from build123d import *

# Parameters (mm, degrees)
F1_DEPTH  = 12
F3_DEPTH  = 25
F4_R      = 1.6
F5_DEPTH  = 12.001
F4_R_2    = 3.25
F6_DEPTH  = 2.5
F8_DEPTH  = 2.5
F9_R      = 1.65
F10_DEPTH = 34.5196429053
F11_R     = 4.99999


# Not quite as in the source:
# - a fillet or chamfer is up to 0.001 mm smaller than in the source, because OpenCascade refuses the exact size


with BuildPart() as f1:
    # F0 (on Right) → F1 (new body)
    with BuildSketch(Plane.YZ):
        Polygon((-19, 5), (-19, -5), (19, -5), (10.3397459622, 0), (14.535244118, 5), align=None)
        Polygon((10.3397459622, 0), (19, -5), (19, 5), (14.535244118, 5), align=None)
        Polygon((19, 5), (19, -5), (41.5633217274, 32.5436371113), (51.2051358727, 44.0343037581), (48.9070025433, 45.9626665871), (14.535244118, 5), align=None)
    extrude(amount=F1_DEPTH)

    # F2 (on face) → F3 (cut)
    with BuildSketch(Plane.XY.offset(5)):
        with BuildLine():
            ThreePointArc((8.4, -10.2369316877), (8.6239283527, -9.6363961031), (8.7, -9))
            ThreePointArc((8.7, -9), (5.3636038969, -6.3760716473), (3.6, -10.2369316877))
            Line((3.6, -10.2369316877), (8.4, -10.2369316877))
        make_face()
        with BuildLine():
            Line((8.4, -10.2369316877), (3.6, -10.2369316877))
            ThreePointArc((3.6, -10.2369316877), (6, -11.7), (8.4, -10.2369316877))
        make_face()
        with BuildLine():
            ThreePointArc((8.4, -10.2369316877), (6, -11.7), (3.6, -10.2369316877))
            Line((3.6, -10.2369316877), (3.6, -19))
            Line((3.6, -19), (8.4, -19))
            Line((8.4, -19), (8.4, -10.2369316877))
        make_face()
    extrude(amount=-F3_DEPTH, mode=Mode.SUBTRACT)

    # F4 (on face) → F5 (cut, through all)
    with BuildSketch(Plane.YZ.offset(12)):
        with Locations((-14, 0)):
            Circle(F4_R)
    extrude(amount=-F5_DEPTH, mode=Mode.SUBTRACT)

    # F4 (on face) → F6 (cut)
    with BuildSketch(Plane.YZ.offset(12)):
        with Locations((-14, 0)):
            Circle(F4_R_2)
        with Locations((-14, 0)):
            Circle(F4_R, mode=Mode.SUBTRACT)
    extrude(amount=-F6_DEPTH, mode=Mode.SUBTRACT)

    # F7 (on face) → F8 (cut)
    with BuildSketch(Plane(origin=(0, 0, 0), x_dir=(0, -1, 0), z_dir=(-1, 0, 0))):
        Polygon((11.15, 1.6454482672), (11.15, -1.6454482672), (14, -3.2908965344), (16.85, -1.6454482672), (16.85, 1.6454482672), (14, 3.2908965344), align=None)
    extrude(amount=-F8_DEPTH, mode=Mode.SUBTRACT)

    # F9 (on face) → F10 (cut, through all)
    with BuildSketch(Plane(origin=(0, 6.067612003, -5.0913309939), x_dir=(1, 0, 0), z_dir=(0, -0.7660444431, 0.6427876097))):
        with Locations((6, 59.6462605918)):
            Circle(F9_R)
    extrude(amount=-F10_DEPTH, mode=Mode.SUBTRACT)

    # F11 (radius 5 in the source; OpenCascade refuses exactly that, so slightly less here)
    f11_edges = [f1.edges().sort_by_distance(p)[0] for p in [
        (1.8, -19, 5),
        (10.2, -19, 5),
        (1.8, -19, -5),
        (10.2, -19, -5),
        (12, 50.056069, 44.998485),
        (0, 50.056069, 44.998485),
        (6, 14.535244, 5),
        (6, 19, -5),
    ]]
    fillet(f11_edges, radius=F11_R)


solid = f1.part
CAD build for the part. Positions are in the model's coordinates, mm. A direction names the side the tool comes from. Give positions to 0.01 mm unless a question says otherwise; leave off trailing zeros. Order: outer loops, then holes, each group sorted by start corner. A loop starts at its lowest first (then second) coordinate and runs counter-clockwise, first axis right, second up. Notation, with made-up numbers: (39, 76) - (49, 76) arc R14 cw to (49, 103) - close; hole circle Ø3 at (47.5, 87). An arc over 180 degrees is marked (long way). Answer in a Markdown table with one row per item.
1. Probe probe 1 along X at (y, z) = (-9, 2.25); probe 2 along Z at (x, y) = (8.9, -14); probe 3 along Z at (x, y) = (9.75, -3). List the from-to ranges inside material, lowest first. Write a range as [from, to].
Data:
| item | result |
|---|---|
| probe 1 | x = [0, 3.3], [8.7, 12] |
| probe 2 | z = [-5, -1.6], [1.6, 5] |
| probe 3 | z = [-5, 5] |
2. Flat gauge pins, fed straight in: pin 1 (1.2 mm diameter, centred on x = 1.5, z = 1, fed in from +Y); pin 2 (2 mm diameter, centred on y = 43, z = 32, fed in from +X); pin 3 (6 mm diameter, centred on x = 10, z = 28.5, fed in from +Y); pin 4 (5 mm diameter, centred on y = -14, z = 0, fed in from -X). Where does each tip first touch, or does it go through?
Data:
| item | result |
|---|---|
| pin 1 | stops at y = 22.97 |
| pin 2 | passes through |
| pin 3 | stops at y = 40.94 |
| pin 4 | stops at x = 2.5 |
3. Saw through at B-B, the plane y = 26. Give the cut face in (x, z), plus the area to 3 significant figures.
Data:
| item | result |
|---|---|
| outline | (0, 6.65) - (12, 6.65) - (12, 18.66) - (0, 18.66) - close |
| area | 144 mm² |
4. Tool access for faces 1 (the cylindrical face through (10.768, -17.247, 0.143)), 2 (the flat face through (6, -1, 5)), 3 (the flat face through (1.232, -12.595, 2.48)): list every direction of +Z, -Z, +X, -X, +Y, -Y with a clear straight run to the whole face (end or side of a thin tool).
Data:
| item | result |
|---|---|
| face 1 | +X |
| face 2 | +Z, +X, -X, -Y |
| face 3 | -X |
5. Saw through at C-C, the plane z = 20.5. Give the cut face in (x, y).
Data:
| item | result |
|---|---|
| outline | (0, 27.54) - (12, 27.54) - (12, 34.33) - (0, 34.33) - close |
6. Pull direction Z, two halves, no side cores. Call faces 4 (the cylindrical face through (2, -18, 3)), 5 (the flat face through (1.232, -15.405, -2.48)), 6 (the cylindrical face through (10, -17, -4)): pulls with the +Z half, pulls with the -Z half, needs draft (parallel to the pull), parting line crosses it, or undercut.
Data:
| item | result |
|---|---|
| face 4 | pulls with the +Z half |
| face 5 | undercut |
| face 6 | pulls with the -Z half |
7. Saw through at A-A, the plane x = 6. Give the cut face in (y, z).
Data:
| item | result |
|---|---|
| outline | (-6.3, -5) - (16.17, -5) arc R5 ccw to (20.46, -2.58) - (41.56, 32.54) - (45.65, 37.41) - (43.35, 39.34) - (16.03, 6.79) arc R5 cw to (12.2, 5) - (-6.3, 5) - close; (45.47, 41.86) - (47.77, 39.94) - (51.21, 44.03) - (48.91, 45.96) - close |
